```python
from build123d import *

# Parameters (mm, degrees)
SKETCH1_R           = 3.75
BOSS_EXTRUDE1_DEPTH = 32
SKETCH2_W           = 1
SKETCH2_H           = 5.5


with BuildPart() as part:
    # Sketch1 → Boss-Extrude1 (new body)
    with BuildSketch(Plane.XY):
        Circle(SKETCH1_R)
    extrude(amount=BOSS_EXTRUDE1_DEPTH)

    # Sketch2 → Revolve1 (revolve)
    with BuildSketch(Plane(origin=(0, 0, 0), x_dir=(1, 0, 0), z_dir=(0, 1, 0))):
        with Locations((4.25, -26.25)):
            Rectangle(SKETCH2_W, SKETCH2_H)
        with Locations((4.25, -5.75)):
            Rectangle(SKETCH2_W, SKETCH2_H)
    revolve(axis=Axis((0, 0, 0), (0, 0, 1)))


solid = part.part
```
Check sheet for the modelled part. Datum: model origin and axes. Units: mm. A direction names the side the tool comes from. Round coordinates to 2 decimals unless told otherwise and drop trailing zeros. Loops run counter-clockwise (first coordinate to the right, second up) from the corner with the lowest first, then second, coordinate; pieces in that order, holes last. Notation, with made-up numbers: (8.25, -1) -> (21.25, -1) arc R19 cw to (21.25, 24) -> close; hole circle Ø11 at (21.5, -18). An arc over 180 degrees is marked (long way). Answer in a Markdown table with one row per item.
Q1. Sectioned sample at A-A on y = 0. Enter the section's corners in (x, z).
Data:
| item | result |
|---|---|
| outline | (-4.75, 3) -> (-3.75, 3) -> (-3.75, 0) -> (3.75, 0) -> (3.75, 3) -> (4.75, 3) -> (4.75, 8.5) -> (3.75, 8.5) -> (3.75, 23.5) -> (4.75, 23.5) -> (4.75, 29) -> (3.75, 29) -> (3.75, 32) -> (-3.75, 32) -> (-3.75, 29) -> (-4.75, 29) -> (-4.75, 23.5) -> (-3.75, 23.5) -> (-3.75, 8.5) -> (-4.75, 8.5) -> close |
Q2. Thickness scan on L1, parallel to Z at x = 2.75, y = 3; L2, parallel to X at y = 0.25, z = 7; L3, parallel to Y at x = -0.25, z = 30. Record the ranges inside material, lowest first.
Data:
| item | result |
|---|---|
| L1 | z = 3 to 8.5, 23.5 to 29 |
| L2 | x = -4.74 to 4.74 |
| L3 | y = -3.74 to 3.74 |
Q3. Set-up check for faces 4 (the face through (4, -1, 8.5)), 5 (the face through (4, -1, 29)), 6 (the face through (4, -1, 3)): record each of +Z, -Z, +X, -X, +Y, -Y from which the full face is reachable in a straight line by a thin tool's end or side.
Data:
| item | result |
|---|---|
| face 4 | none |
| face 5 | +Z |
| face 6 | -Z |
Q4. Release check for a two-part mould opening along Z. For faces 1 (the face through (0, 0, 32)), 2 (the face through (-3.746, 0.165, 15.895)), 3 (the face through (2.192, -4.214, 26.212)) record: released by +Z, released by -Z, zero draft, split by the parting line, or undercut.
Data:
| item | result |
|---|---|
| face 1 | released by +Z |
| face 2 | undercut |
| face 3 | zero draft |
Q5. Go/stop test with flat-tipped pins: P1, Ø2, axis at x = -3, z = 5, coming from the -Y side; P2, Ø3, axis at x = 3.5, z = 19, coming from the +Y side; P3, Ø1.5, axis at x = 1, z = 12.5, coming from the +Y side. Record where each tip stops, or that it passes through.
Data:
| item | result |
|---|---|
| P1 | stops at y = -4.31 |
| P2 | stops at y = 3.17 |
| P3 | stops at y = 3.74 |
Q6. Sectioned sample at C-C on z = 11.5. Enter the section's corners in (x, y).
Data:
| item | result |
|---|---|
| outline | circle Ø7.5 at (0, 0) |
